from build123d import *

# Parameters (mm, degrees)
SKETCH1_W              = 17.78
SKETCH1_H              = 17.78
EXTRUSION1_DEPTH       = 1.27
EXTRUSION2_DEPTH       = 1.27
SKETCH3_R              = 1.5875
EXTRUSION3_DEPTH       = 0.381
HOLE1_D                = 0.5334
HOLE2_D                = 0.7874
EXTRUSION4_START       = -0.635
EXTRUSION4_OUTLINE_R   = 0.2667
EXTRUSION4_OUTLINE_R_2 = 0.3937
EXTRUSION4_DEPTH       = 0.635
FILLET1_R              = 2.54


# Read off the part's stored shape, not the designer's step: Extrusion4
with BuildPart() as part:
    # Sketch1 → Extrusion1 (new body)
    with BuildSketch(Plane.XY):
        Polygon((12.7, 11.43), (11.43, 12.7), (-11.43, 12.7), (-12.7, 11.43), (-12.7, -11.43), (-11.43, -12.7), (11.43, -12.7), (12.7, -11.43), align=None)
        with Locations((0.037350374, -0.075564582)):
            Rectangle(SKETCH1_W, SKETCH1_H, mode=Mode.SUBTRACT)
    extrude(amount=EXTRUSION1_DEPTH)

    # Sketch2 → Extrusion2 (add)
    with BuildSketch(Plane.XY.offset(1.27)):
        with BuildLine():
            ThreePointArc((1.800535754, -12.7), (9.070058682, -9.070058682), (12.7, -1.800535754))
            Line((12.7, -1.800535754), (12.7, -11.43))
            Line((12.7, -11.43), (11.43, -12.7))
            Line((11.43, -12.7), (1.800535754, -12.7))
        make_face()
        with BuildLine():
            ThreePointArc((-12.7, -1.800535754), (-9.070058682, -9.070058682), (-1.800535754, -12.7))
            Line((-1.800535754, -12.7), (-11.43, -12.7))
            Line((-11.43, -12.7), (-12.7, -11.43))
            Line((-12.7, -11.43), (-12.7, -1.800535754))
        make_face()
        with BuildLine():
            ThreePointArc((-1.800535754, 12.7), (-9.070058682, 9.070058682), (-12.7, 1.800535754))
            Line((-12.7, 1.800535754), (-12.7, 11.43))
            Line((-12.7, 11.43), (-11.43, 12.7))
            Line((-11.43, 12.7), (-1.800535754, 12.7))
        make_face()
        with BuildLine():
            ThreePointArc((12.7, 1.800535754), (9.070058682, 9.070058682), (1.800535754, 12.7))
            Line((1.800535754, 12.7), (11.43, 12.7))
            Line((11.43, 12.7), (12.7, 11.43))
            Line((12.7, 11.43), (12.7, 1.800535754))
        make_face()
    extrude(amount=EXTRUSION2_DEPTH)

    # Sketch3 → Extrusion3 (cut)
    with BuildSketch(Plane(origin=(0, 0, 0), x_dir=(-1, 0, 0), z_dir=(0, 0, -1))):
        with Locations((-10.414, 10.414)):
            Circle(SKETCH3_R)
    extrude(amount=-EXTRUSION3_DEPTH, mode=Mode.SUBTRACT)

    # Hole1 (through all)
    with Locations(Plane(origin=(0, 0, 0.381), x_dir=(-1, 0, 0), z_dir=(0, 0, -1))):
        with Locations((-10.414, 11.43), (-11.29388181, 9.906), (-9.53411819, 9.906)):
            Hole(HOLE1_D / 2)

    # Hole2 (through all)
    with Locations(Plane(origin=(0, 0, 0.381), x_dir=(-1, 0, 0), z_dir=(0, 0, -1))):
        with Locations((-10.414, 10.414)):
            Hole(HOLE2_D / 2)

    # Extrusion4 outline → Extrusion4 (cut)
    with BuildSketch(Plane.XY.offset(2.54).offset(EXTRUSION4_START)):
        with BuildLine():
            ThreePointArc((11.518713485, 9.273649455), (11.536532015, 11.536532015), (9.27379199, 11.518573195))
            Line((9.27379199, 11.518573195), (7.877795, 10.12285903))
            ThreePointArc((7.877795, 10.12285903), (9.070058682, 9.070058682), (10.12285903, 7.877795))
            Line((10.12285903, 7.877795), (11.518713485, 9.273649455))
        make_face()
        with Locations((9.53411819, 9.906)):
            Circle(EXTRUSION4_OUTLINE_R, mode=Mode.SUBTRACT)
        with Locations((11.29388181, 9.906)):
            Circle(EXTRUSION4_OUTLINE_R, mode=Mode.SUBTRACT)
        with Locations((10.414, 10.414)):
            Circle(EXTRUSION4_OUTLINE_R_2, mode=Mode.SUBTRACT)
        with Locations((10.414, 11.43)):
            Circle(EXTRUSION4_OUTLINE_R, mode=Mode.SUBTRACT)
    extrude(amount=EXTRUSION4_DEPTH, mode=Mode.SUBTRACT)

    # Fillet1
    fillet1_edges = [part.edges().sort_by_distance(p)[0] for p in [
        (8.927350374, -8.965564582, 0.635),
        (8.927350374, 8.814435418, 0.635),
        (-8.852649626, 8.814435418, 0.635),
        (-8.852649626, -8.965564582, 0.635),
    ]]
    fillet(fillet1_edges, radius=FILLET1_R)


solid = part.part
Geometry: final body of the model. Coordinates: model frame, mm. A direction names the side the tool comes from. Round coordinates to 2 decimals unless told otherwise and drop trailing zeros. Loops run counter-clockwise (first coordinate to the right, second up) from the corner with the lowest first, then second, coordinate; pieces in that order, holes last. Notation, with made-up numbers: (30.25, 78) -> (72.25, 78) arc R29 ccw to (72.25, 113) -> close; hole circle Ø2 at (1.25, 54.5). An arc over 180 degrees is marked (long way). One line per question, with ' | ' between items. Start each with the question number.
1. Set-up query: faces 5 (the face through (10, 10, 0.381)), 6 (the face through (8.586, 10.83, 2.218)), 7 (the face through (0, -8.966, 1)), 8 (the face through (12.07, 12.06, 1.25)). Return all of +Z, -Z, +X, -X, +Y, -Y with unobstructed straight access to the full face (end or side cutting, diameter ignored); none if empty.
2. Section B-B on y = -9.75. Output: boundary loops of the cut face in (x, z).
3. Mould query, pull axis X, two halves, no side actions, for faces 1 (the face through (9.15, 8.99, 1.75)), 2 (the face through (0, -12.7, 1)), 3 (the face through (-12.06, 12.07, 1.25)), 4 (the face through (-8.853, 0, 1)). Classes: pulls with the +X half, pulls with the -X half, needs draft (parallel to the pull), parting line crosses it, or undercut.
4. Section C-C on x = -10.25. Output: boundary loops of the cut face in (y, z).
5. Section D-D on x = 7.5. Output: boundary loops of the cut face in (y, z), and give its area (3 significant figures).
6. Line query: line 1 along Y through (x, z) = (2.5, 0.15); line 2 along Y through (x, z) = (10.25, 1.15); line 3 along X through (y, z) = (-0.25, 0.7). Output: solid intervals per line, ascending. Write a range as [from, to].
7. Contact query for flat-ended pins moving along their axis: pin 1 (5 mm diameter, centred on x = 10, y = 9.5, fed in from -Z); pin 2 (1.9 mm diameter, centred on x = 10.414, y = 10.414, fed in from +Z) (3 decimals); pin 3 (5 mm diameter, centred on x = -2, y = 5.5, fed in from -Z); pin 4 (12.5 mm diameter, centred on x = -4, y = 4, fed in from +Z). Output: stop coordinate, or through.
8. Section A-A on x = -3. Output: boundary loops of the cut face in (y, z), and give its area (3 significant figures).
Returned:
1) face 5: -Z | face 6: +Z | face 7: +Z, -Z | face 8: +Z, -Z, +X, +Y
2) outline: (-12.7, 0) -> (12.7, 0) -> (12.7, 2.54) -> (8.33, 2.54) -> (8.33, 1.27) -> (-8.33, 1.27) -> (-8.33, 2.54) -> (-12.7, 2.54) -> close
3) face 1: undercut | face 2: needs draft | face 3: pulls with the -X half | face 4: undercut
4) outline: (-12.7, 0) -> (12.7, 0) -> (12.7, 2.54) -> (7.71, 2.54) -> (7.71, 1.27) -> (-7.71, 1.27) -> (-7.71, 2.54) -> (-12.7, 2.54) -> close
5) outline: (-12.7, 0) -> (-8.71, 0) -> (-8.71, 1.27) -> (-10.41, 1.27) -> (-10.41, 2.54) -> (-12.7, 2.54) -> close; (8.56, 0) -> (12.7, 0) -> (12.7, 2.54) -> (10.41, 2.54) -> (10.41, 1.27) -> (8.56, 1.27) -> close | area: 16.2 mm2
6) line 1: y = [-12.7, -8.97], [8.81, 12.7] | line 2: y = [-12.7, 10.06], [10.77, 11.22], [11.64, 12.7] | line 3: x = [-12.7, -8.85], [8.93, 12.7]
7) pin 1: stops at z = 0 | pin 2: stops at z = 1.905 | pin 3: passes through | pin 4: stops at z = 1.27
8) outline: (-12.7, 0) -> (-8.97, 0) -> (-8.97, 1.27) -> (-12.47, 1.27) -> (-12.47, 2.54) -> (-12.7, 2.54) -> close; (8.81, 0) -> (12.7, 0) -> (12.7, 2.54) -> (12.47, 2.54) -> (12.47, 1.27) -> (8.81, 1.27) -> close | area: 10.3 mm2
